Geometry: final body of the model. Coordinates: model frame, mm. Give positions to 0.01 mm unless a question says otherwise; leave off trailing zeros. Order: outer loops, then holes, each group sorted by start corner. A loop starts at its lowest first (then second) coordinate and runs counter-clockwise, first axis right, second up. Notation, with made-up numbers: (-6, -26.75) -> (53, -26.75) arc R17 cw to (53, -5.75) -> close; hole circle Ø1 at (37, 9). An arc over 180 degrees is marked (long way). One line per item, written item: value. Start each with the question number.
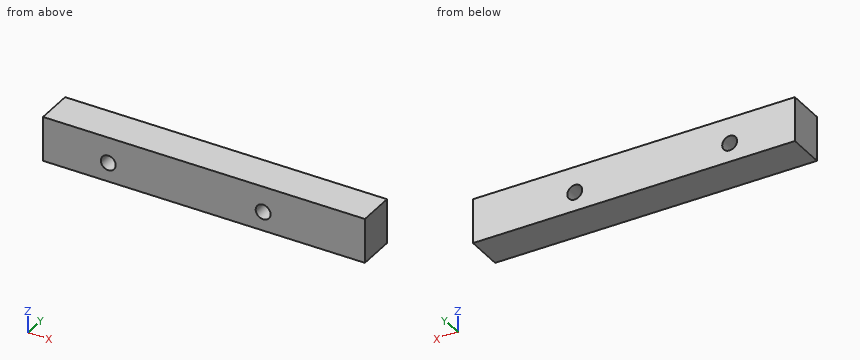
```python
from build123d import *

# Parameters (mm, degrees)
F0_W          = 130
F0_H          = 18
F0_R          = 3
F1_DEPTH      = 7.5
F2_R          = 3
F3_DEPTH      = 7.501
F3_DEPTH_BACK = 25


with BuildPart() as f1:
    # F0 (on Front) → F1 (new body, symmetric)
    with BuildSketch(Plane.XZ):
        with Locations((0, -9)):
            Rectangle(F0_W, F0_H)
        with Locations((-32.9453274608, -9.836692363)):
            Circle(F0_R, mode=Mode.SUBTRACT)
        with Locations((41.1642305553, -9.836692363)):
            Circle(F0_R, mode=Mode.SUBTRACT)
        with Locations((-32.9453274608, -9.836692363)):
            Circle(F0_R)
        with Locations((41.1642305553, -9.836692363)):
            Circle(F0_R)
    extrude(amount=F1_DEPTH, both=True)

    # F2 (on Front) → F3 (cut, two sides)
    with BuildSketch(Plane.XZ) as f3_sk:
        with Locations((-38.6426560581, -10.3746056557)):
            Circle(F2_R)
        with Locations((23.9025931805, -10.3746056557)):
            Circle(F2_R)
    extrude(amount=-F3_DEPTH, mode=Mode.SUBTRACT)
    extrude(f3_sk.sketch, amount=F3_DEPTH_BACK, mode=Mode.SUBTRACT)


solid = f1.part
```
1. Cut plane A-A, the plane z = -12.25. Return loops of the section in (x, y), then the cut area to 3 significant figures.
2. Material intervals for L1, parallel to X at y = 2.5, z = -10.25; L2, parallel to X at y = 5, z = -10; L3, parallel to Z at x = -36.5, y = 6.25, sorted ascending. Write a range as [from, to].
3. Cut plane B-B, the plane y = 3.25. Return loops of the section in (x, z).
4. Pin query (flat end, axial travel): P1, Ø2, axis at x = 5.5, y = -5.5, coming from the +Z side; P2, Ø3.5, axis at x = -38.64, z = -10.37, coming from the +Y side. Return the tip coordinate at first contact, or that it passes through.
Answers follow:
1. outline: (-65, -7.5) -> (-40.98, -7.5) -> (-40.98, 7.5) -> (-65, 7.5) -> close; (-36.3, -7.5) -> (21.56, -7.5) -> (21.56, 7.5) -> (-36.3, 7.5) -> close; (26.24, -7.5) -> (65, -7.5) -> (65, 7.5) -> (26.24, 7.5) -> close
1. area: 1,810 mm²
2. L1: x = [-65, -41.64], [-35.65, 20.91], [26.9, 65]
2. L2: x = [-65, -41.62], [-35.67, 20.93], [26.88, 65]
2. L3: z = [-18, -12.47], [-8.27, 0]
3. outline: (-65, -18) -> (65, -18) -> (65, 0) -> (-65, 0) -> close; hole circle Ø6 at (-38.64, -10.37); hole circle Ø6 at (23.9, -10.37)
4. P1: stops at z = 0
4. P2: passes through
